Geometry: see drawing. Coordinates: mm, zero at the bounding-box minimum. A direction names the side the tool comes from. Give positions to 0.01 mm unless a question says otherwise; leave off trailing zeros. Loops run counter-clockwise (first coordinate to the right, second up) from the corner with the lowest first, then second, coordinate; pieces in that order, holes last. Notation, with made-up numbers: (-29, -29.5) -> (-5, -29.5) arc R16 ccw to (-5, -23.5) -> close; hole circle Ø9 at (49, 66). An arc over 180 degrees is marked (long way). Return JSON: item names as keys, results as strings. Group by question number.
(1) Cut plane D-D on z = 19. Return loops of the section in (x, y), then the cut area to 3 significant figures.
(2) Draft query along X for the marked faces 1, 2 and 3. Return one class per face: released by +X, released by -X, zero draft, split by the parting line, or undercut.
(3) Access query for the marked faces 4, 5 and 6. Directions: +Z, -Z, +X, -X, +Y, -Y. A direction counts if a zero-diameter tool reaches every point of the face in a straight line with its end or side. Return the directions, or none.
(4) Cut plane B-B on z = 11.75. Return loops of the section in (x, y).
(5) Cut plane C-C on y = 12. Return loops of the section in (x, z), then the cut area to 3 significant figures.
(6) Ray query, line 1 (Z direction, x = 8.5, y = 3.75); line 2 (X direction, y = 4.25, z = 17); line 3 (Y direction, x = 5.5, z = 5.75). Return the intervals inside material, ascending. Write a range as from..to.
(7) Pin query (flat end, axial travel): pin 1 (5 mm diameter, centred on x = 15, z = 12.5, fed in from +Y); pin 2 (0.8 mm diameter, centred on y = 0.5, z = 18.5, fed in from +X); pin 3 (0.8 mm diameter, centred on x = 9.5, z = 0.5, fed in from +Y). Return the tip coordinate at first contact, or that it passes through.
(8) Cut plane A-A on x = 8.5. Give the number of separate pieces and of enclosed holes in the cut face, then the cut area to 3 significant figures.
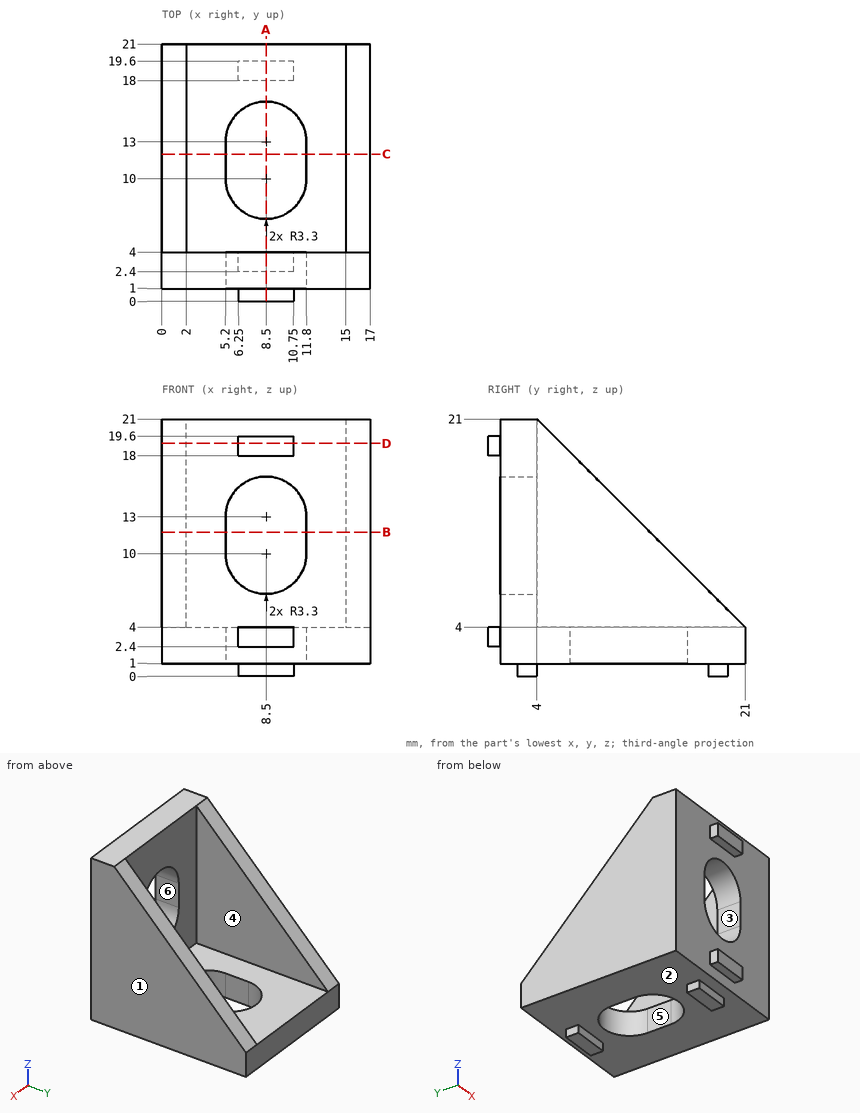
Answers:
{
 "1": {"outline": "(0, 1) -> (6.25, 1) -> (6.25, 0) -> (10.75, 0) -> (10.75, 1) -> (17, 1) -> (17, 6) -> (15, 6) -> (15, 4) -> (2, 4) -> (2, 6) -> (0, 6) -> close", "area": "63.5 mm²"},
 "2": {"face 1": "released by +X", "face 2": "zero draft", "face 3": "undercut"},
 "3": {"face 4": "+Z, +Y", "face 5": "+Z, -Z", "face 6": "+Y, -Y"},
 "4": {"outline": "(0, 1) -> (5.2, 1) -> (5.2, 4) -> (2, 4) -> (2, 13.25) -> (0, 13.25) -> close; (11.8, 1) -> (17, 1) -> (17, 13.25) -> (15, 13.25) -> (15, 4) -> (11.8, 4) -> close"},
 "5": {"outline": "(0, 1) -> (5.2, 1) -> (5.2, 4) -> (2, 4) -> (2, 13) -> (0, 13) -> close; (11.8, 1) -> (17, 1) -> (17, 13) -> (15, 13) -> (15, 4) -> (11.8, 4) -> close", "area": "67.2 mm²"},
 "6": {"line 1": "0..6.7, 16.3..21", "line 2": "0..2, 15..17", "line 3": "1..4"},
 "7": {"pin 1": "y = 15", "pin 2": "x = 10.75", "pin 3": "y = 19.6"},
 "8": {"separate pieces": "3", "enclosed holes": "0", "area": "59.8 mm²"}
}
